Verification items for the finished model (mm, model axes). A direction names the side the tool comes from. Give positions to 0.01 mm unless a question says otherwise; leave off trailing zeros. Order: outer loops, then holes, each group sorted by start corner. A loop starts at its lowest first (then second) coordinate and runs counter-clockwise, first axis right, second up. Notation, with made-up numbers: (65.5, -13) -> (77.5, -13) arc R26 ccw to (77.5, 13) -> close; hole circle Ø11 at (35, 26.5). An arc over 180 degrees is marked (long way). One line per question, with ' | ' between items. Start each with the question number.
Q1. Section check B-B on x = 0. Record the cut outline in (y, z).
Q2. Go/stop test with flat-tipped pins: pin 1 (0.5 mm diameter, centred on y = 0.5, z = 0.5, fed in from -X); pin 2 (3 mm diameter, centred on x = 2, z = -0.5, fed in from +Y); pin 3 (0.5 mm diameter, centred on x = 1, z = 0.5, fed in from +Y). Record where each tip stops, or that it passes through.
Q3. Section check A-A on z = 0.35. Record the cut outline in (x, y), plus the area to 3 significant figures.
Q4. Section check D-D on z = -4.45. Record the cut outline in (x, y), plus the area to 3 significant figures.
Q5. Access from +Z, -Z, +X, -X, +Y, -Y to the whole of each face (thin tool, end or side, straight path). Record for faces 4 (the flat face through (0, 0, -5)), 5 (the cylindrical face through (1.5, -0.07, -2.46)).
Q6. Material ranges on probe 1 along Z at (x, y) = (-0.4, -1.9); probe 2 along X at (y, z) = (0.35, 0.3); probe 3 along Y at (x, z) = (-1.05, -0.65), recorded low to high. Write a range as [from, to].
Q7. Mould release check, pull along Y, two halves, no side actions. Record for faces 1 (the flat face through (1.2, -1.2, 0)), 2 (the cylindrical face through (-0.596, 2.685, 0.345)), 3 (the flat face through (0, 0, 0.2)): released by +Y, released by -Y, zero draft, split by the parting line, or undercut.
Autodesk Inventor part; units mm, degrees
ref_plane "YZ Plane" through (0, 0, 0) normal (1, 0, 0) x (0, 1, 0)
ref_plane "XZ Plane" through (0, 0, 0) normal (0, 1, 0) x (-1, 0, 0)
ref_plane "XY Plane" through (0, 0, 0) normal (0, 0, 1) x (1, 0, 0)
sketch "スケッチ1" plane through (0, 0, 0) normal (0, 0, 1) x (1, 0, 0)
  circle A0 centre (0, 0) radius 2.75
  dimension "d0" = 5.5
extrude "押し出し1" add sketch "スケッチ1" along normal blind 0.7
sketch "スケッチ2" plane through (0, 0, 0) normal (0, 0, -1) x (-1, 0, 0)
  circle A0 centre (0, 0) radius 1.5
  dimension "d3" = 3
extrude "押し出し2" add sketch "スケッチ2" along normal blind 5
sketch "スケッチ3" plane through (0, 0, 0.7) normal (0, 0, 1) x (1, 0, 0)
  line L0 (-1.25, 0.25) -> (1.25, 0.25)
  line L1 (1.25, 0.25) -> (1.25, -0.25)
  line L2 (1.25, -0.25) -> (-1.25, -0.25)
  line L3 (-1.25, -0.25) -> (-1.25, 0.25)
  line L4 (-0.25, 1.25) -> (0.25, 1.25)
  line L5 (0.25, 1.25) -> (0.25, -1.25)
  line L6 (0.25, -1.25) -> (-0.25, -1.25)
  line L7 (-0.25, -1.25) -> (-0.25, 1.25)
  line L8 (0, 0) -> (0, 1.7976)
  line L9 (0, 0) -> (2.75, 0)
  circle A0 centre (0, 0) radius 2.75
  point P0 (-0.25, 0.25)
  point P1 (-0.25, -0.25)
  point P2 (0.25, -0.25)
  point P3 (0.25, 0.25)
  dimension "d6" = 0.5
  dimension "d7" = 0.5
  dimension "d8" = 2.5
  dimension "d9" = 2.5
extrude "押し出し3" cut sketch "スケッチ3" against normal blind 0.5 contours L0 L7 L2 L3 | L7 L4 L8 L0 | L0 L8 L9 L5 L2 L7 | L8 L4 L5 L0 | L0 L5 L9 L8 | L2 L5 L6 L7 | L0 L1 L9 L5 | L5 L9 L1 L2
properties part number "CSPELH-SUS-M3-5"
Filled in:
1) outline: (-2.75, 0) -> (-1.5, 0) -> (-1.5, -5) -> (1.5, -5) -> (1.5, 0) -> (2.75, 0) -> (2.75, 0.7) -> (1.25, 0.7) -> (1.25, 0.2) -> (-1.25, 0.2) -> (-1.25, 0.7) -> (-2.75, 0.7) -> close
2) pin 1: x = -2.74 | pin 2: y = 2.69 | pin 3: y = 2.65
3) outline: circle Ø5.5 at (0, 0); hole (-1.25, -0.25) -> (-0.25, -0.25) -> (-0.25, -1.25) -> (0.25, -1.25) -> (0.25, -0.25) -> (1.25, -0.25) -> (1.25, 0.25) -> (0.25, 0.25) -> (0.25, 1.25) -> (-0.25, 1.25) -> (-0.25, 0.25) -> (-1.25, 0.25) -> close | area: 21.5 mm²
4) outline: circle Ø3 at (0, 0) | area: 7.07 mm²
5) face 4: -Z, +X, -X, +Y, -Y | face 5: -Z
6) probe 1: [0, 0.7] | probe 2: [-2.73, -0.25], [0.25, 2.73] | probe 3: [-1.07, 1.07]
7) face 1: zero draft | face 2: split by the parting line | face 3: undercut
